CAD build for the part. Positions are in the model's coordinates, mm. A direction names the side the tool comes from. Give positions to 0.01 mm unless a question says otherwise; leave off trailing zeros. Loops run counter-clockwise (first coordinate to the right, second up) from the corner with the lowest first, then second, coordinate; pieces in that order, holes last. Notation, with made-up numbers: (43.5, 65.25) -> (55.5, 65.25) arc R18 cw to (55.5, 93.25) -> close; hole circle Ø1 at (41.25, 46). An arc over 180 degrees is marked (long way). Write each question's results on one line, items separated by ' | '. Start each with the question number.
Autodesk Inventor part; units mm, degrees
ref_plane "Work Plane15" through (0, 0, 83) normal (0, 0, 1) x (1, 0, 0)
ref_plane "YZ Plane" through (0, 0, 0) normal (1, 0, 0) x (0, 1, 0)
ref_plane "XZ Plane" through (0, 0, 0) normal (0, 1, 0) x (-1, 0, 0)
ref_plane "Work Plane15" through (0, 0, 83) normal (0, 0, 1) x (1, 0, 0)
sketch "Sketch35" plane through (0, 0, 83) normal (0, 0, 1) x (1, 0, 0)
  line L0 (-53.15, -19.2) -> (-22.85, -19.2)
  line L1 (-22.85, -19.2) -> (-22.85, -26.8)
  line L2 (-22.85, -26.8) -> (-53.15, -26.8)
  line L3 (-53.15, -26.8) -> (-53.15, -19.2)
  line L4 (-53.15, -26.8) -> (-22.85, -19.2) construction
  line L5 (-22.85, -26.8) -> (-53.15, -19.2) construction
  line L6 (-53.15, -23) -> (-49.35, -23) construction
  arc A0 (-49.35, -19.2) -> (-53.15, -23) centre (-49.35, -23) ccw
  arc A1 (-53.15, -23) -> (-49.35, -26.8) centre (-49.35, -23) ccw
  line L7 (-22.85, -23) -> (-26.65, -23) construction
  arc A2 (-22.85, -23) -> (-26.65, -19.2) centre (-26.65, -23) ccw
  arc A3 (-26.65, -26.8) -> (-22.85, -23) centre (-26.65, -23) ccw
  line L8 (-38, -26.8) -> (-38, -23)
  line L9 (-38, -26.8) -> (-34.2, -26.8) construction
  line L10 (-28, 6.8) -> (28, 6.8)
  line L11 (28, 6.8) -> (28, -6.8)
  line L12 (28, -6.8) -> (-28, -6.8)
  line L13 (-28, -6.8) -> (-28, 6.8)
  line L14 (-11.3, -22) -> (-6.85, -22) construction
  line L15 (3, -17.55) -> (3, -26.45)
  line L16 (-11.5, -17.5) -> (17.5, -17.5)
  line L17 (17.5, -17.5) -> (17.5, -26.5)
  line L18 (17.5, -26.5) -> (-11.5, -26.5)
  line L19 (-11.5, -26.5) -> (-11.5, -17.5)
  line L20 (-11.5, -22) -> (-7, -22)
  arc A4 (-7, -17.5) -> (-7, -26.5) centre (-7, -22) ccw
  arc A5 (13, -26.5) -> (13, -17.5) centre (13, -22) ccw
  line L21 (-15.1, 4.5) -> (15.1, 4.5)
  line L22 (15.1, 4.5) -> (15.1, -4.5)
  line L23 (15.1, -4.5) -> (-15.1, -4.5)
  line L24 (-15.1, -4.5) -> (-15.1, 4.5)
  line L25 (-15.1, 0) -> (-10.6, 0)
  arc A6 (-10.6, 4.5) -> (-10.6, -4.5) centre (-10.6, 0) ccw
  arc A7 (10.6, -4.5) -> (10.6, 4.5) centre (10.6, 0) ccw
  line L26 (0, 4.5) -> (0, -4.5)
  point P0 (0, 0)
  point P1 (69, 73)
  point P2 (-22.85, -23)
  point P3 (-22.85, -23)
  point P4 (-26.65, -26.8)
  point P5 (-26.65, -19.2)
  point P6 (13, -26.5)
  point P7 (13, -17.5)
  point P8 (0, 0)
  dimension "d253" = 7.6
  dimension "d265" = 3.8
  dimension "d316" = 3.8
  dimension "d317" = 90
  dimension "d359" = 29
  dimension "d360" = 9
  dimension "d361" = 4.5
  dimension "d362" = 30.2
  dimension "d363" = 9
  dimension "d364" = 4.5
  dimension "d365" = 56
  dimension "d366" = 13.6
  dimension "d367" = 2.3
  dimension "d368" = 12.9
extrude "Extrusion25" add sketch "Sketch35" against normal blind 7.7 contours L10 L11 L12 L13 | L21 A6 L24 | A6 L23 L24 | L21 L22 A7 | L22 L23 A7
sketch "Sketch46" plane through (0, 0, 83) normal (0, 0, 1) x (1, 0, 0)
  point P0 (0, 0)
  point P1 (-20, 0)
  point P2 (20, 0)
hole "Hole8" at (20, 0, 83) at (-20, 0, 83) direction (0, 0, -1) diameter 4.2 depth 7.7 counterbore diameter 8 counterbore depth 4
sketch "Sketch47" plane through (0, 0, 75.3) normal (0, 0, -1) x (-1, 0, 0)
  line L0 (28, -3) -> (25, -3)
  line L1 (25, -3) -> (25, 3)
  line L2 (25, 3) -> (28, 3)
  line L3 (28, 3) -> (28, -3)
  line L4 (0, 0) -> (0, 11)
  line L5 (-28, -3) -> (-25, -3)
  line L6 (-25, -3) -> (-25, 3)
  line L7 (-25, 3) -> (-28, 3)
  line L8 (-28, 3) -> (-28, -3)
  line L9 (28, -6.8) -> (28, 6.8)
  dimension "d378" = 3
  dimension "d379" = 6
  dimension "d380" = 0
extrude "Extrusion34" add sketch "Sketch47" along normal blind 3
properties part number "cameraModuleEnclosure_3DPrint"
Q1. Which spindle directions (+Z, -Z, +X, -X, +Y, -Y) get a long thin tool onto all of the face, cutting with end or side? Do faces 1 (the face through (-27, -3, 74)), 2 (the face through (26, 3, 74)), 3 (the face through (0, 4.5, 79)). Say none if no direction does.
Q2. Drop flat-ended pins along their axis: pin 1 (0.9 mm diameter, centred on x = 27, z = 74, fed in from +Y); pin 2 (3.5 mm diameter, centred on x = -20, y = 0, fed in from +Z); pin 3 (7 mm diameter, centred on x = -11.5, y = -3, fed in from -Z); pin 4 (5.5 mm diameter, centred on x = 20, y = 0, fed in from +Z). Give the stop position or say it passes through.
Q3. Saw through at B-B, the plane z = 73.75. List the corners of the cut face in (x, y).
Q4. Saw through at D-D, the plane z = 77. List the corners of the cut face in (x, y), then the cut area to 3 significant figures.
Q5. Wall check: L1, parallel to X at y = 0, z = 81.65; L2, parallel to X at y = 0, z = 77.2; L3, parallel to Y at x = 20, z = 78.15. Give the ranges that are in metal, low to high.
Q6. Saw through at C-C, the plane y = 0. List the corners of the cut face in (x, z).
Q7. Saw through at A-A, the plane x = 4.5. List the corners of the cut face in (y, z), then the cut area to 3 significant figures.
Q8. Mould opens along Y. For faces 4 (the face through (22, -2, 79)), 5 (the face through (-25, 0, 74)), 6 (the face through (0, -6.8, 79)) say: pulls with the +Y half, pulls with the -Y half, needs draft (parallel to the pull), parting line crosses it, or undercut.
Answer block:
1) face 1: -Z, +X, -X, -Y | face 2: -Z, +X, -X, +Y | face 3: +Z, -Z
2) pin 1: stops at y = 3 | pin 2: passes through | pin 3: stops at z = 75.3 | pin 4: stops at z = 79
3) outline: (-28, -3) -> (-25, -3) -> (-25, 3) -> (-28, 3) -> close; (25, -3) -> (28, -3) -> (28, 3) -> (25, 3) -> close
4) outline: (-28, -6.8) -> (28, -6.8) -> (28, 6.8) -> (-28, 6.8) -> close; hole circle Ø4.2 at (-20, 0); hole (-10.6, -4.5) -> (10.6, -4.5) arc R4.5 ccw to (10.6, 4.5) -> (-10.6, 4.5) arc R4.5 ccw to start; hole circle Ø4.2 at (20, 0) | area: 479 mm2
5) L1: x = -28 to -24, -16 to -15.1, 15.1 to 16, 24 to 28 | L2: x = -28 to -22.1, -17.9 to -15.1, 15.1 to 17.9, 22.1 to 28 | L3: y = -6.8 to -2.1, 2.1 to 6.8
6) outline: (-28, 72.3) -> (-25, 72.3) -> (-25, 75.3) -> (-22.1, 75.3) -> (-22.1, 79) -> (-24, 79) -> (-24, 83) -> (-28, 83) -> close; (-17.9, 75.3) -> (-15.1, 75.3) -> (-15.1, 83) -> (-16, 83) -> (-16, 79) -> (-17.9, 79) -> close; (15.1, 75.3) -> (17.9, 75.3) -> (17.9, 79) -> (16, 79) -> (16, 83) -> (15.1, 83) -> close; (22.1, 75.3) -> (25, 75.3) -> (25, 72.3) -> (28, 72.3) -> (28, 83) -> (24, 83) -> (24, 79) -> (22.1, 79) -> close
7) outline: (-6.8, 75.3) -> (-4.5, 75.3) -> (-4.5, 83) -> (-6.8, 83) -> close; (4.5, 75.3) -> (6.8, 75.3) -> (6.8, 83) -> (4.5, 83) -> close | area: 35.4 mm2
8) face 4: undercut | face 5: needs draft | face 6: pulls with the -Y half
